Here's the drawing with two shaded views (mm, measured from the low corner). I have some questions. A direction names the side the tool comes from. Give positions to 0.01 mm unless a question says otherwise; leave off trailing zeros. Loops run counter-clockwise (first coordinate to the right, second up) from the corner with the lowest first, then second, coordinate; pieces in that order, holes last. Notation, with made-up numbers: M -21,-31.75 L 19,-31.75 A13 cw 19,-23.75 Z; hole C 28.25,21.5 d8. An arc over 180 degrees is marked long. Use a Markdown table: item, result. Add a question column.
1) Suppose I cut it at D-D on z = 2. List the corners of the cut face in (x, y) for me (3 decimals).
2) Suppose I cut it at C-C on z = 7. List the corners of the cut face in (x, y) for me, and give its area (3 significant figures).
3) If I drill on line 1 along X through (y, z) = (36, 10.25); line 2 along Z through (x, y) = (8, 28.5); line 3 along Y through (x, z) = (38.8, 6), over which ranges is the centre line in solid material (lowest first)? Write a range as [from, to].
4) Suppose I cut it at A-A on y = 30. List the corners of the cut face in (x, z) for me (3 decimals), and give its area (3 significant figures).
5) Which directions (+Z, -Z, +X, -X, +Y, -Y) give clear straight access to the entire face, cutting with the end or side of a thin tool? Please do the marked faces 1, 2 and 3.
6) We'd pull the mould along X, two halves only. Please class the marked faces 4, 5 and 6: +X half, -X half, draft (parallel to the pull), parting line (faces both ways), or undercut.
7) Suppose I cut it at B-B on x = 30. List the corners of the cut face in (y, z) for me.
8) Will these pins go through, and if not, where does the flat tip stop? pin 1 Ø13.5 at (x, y) = (38.8, 30) entering from +Z; pin 2 Ø1 at (x, z) = (42.5, 4.5) entering from -Y; pin 3 Ø1.5 at (x, y) = (8, 29.5) entering from -Z.
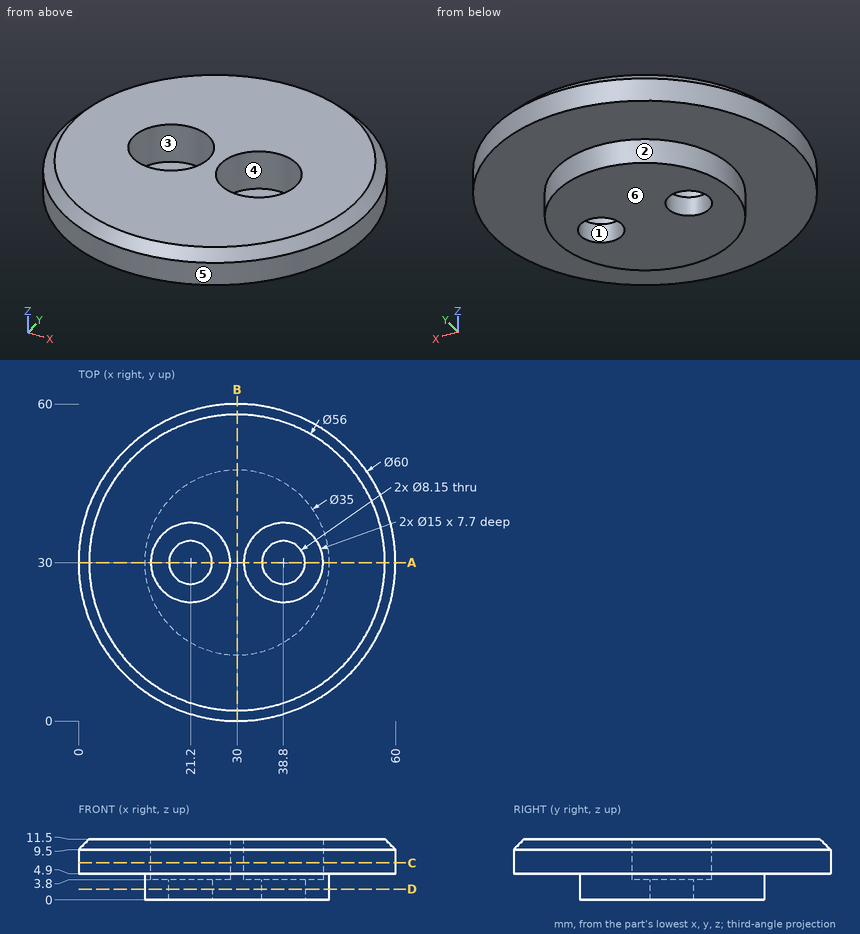
Answer block:
| question | item | result |
|---|---|---|
| 1 | outline | C 30,30 d35; hole C 21.2,30 d8.15; hole C 38.8,30 d8.15 |
| 2 | outline | C 30,30 d60; hole C 21.2,30 d15; hole C 38.8,30 d15 |
| 2 | area | 2,470 mm^2 |
| 3 | line 1 | x = [1.37, 16.7], [25.7, 34.3], [43.3, 58.63] |
| 3 | line 2 | z = [4.9, 11.5] |
| 3 | line 3 | y = [1.32, 22.5], [37.5, 58.68] |
| 4 | outline | M 0,4.9 L 12.5,4.9 L 12.5,0 L 17.125,0 L 17.125,3.8 L 13.7,3.8 L 13.7,11.5 L 2,11.5 L 0,9.5 Z; M 25.275,0 L 34.725,0 L 34.725,3.8 L 31.3,3.8 L 31.3,11.5 L 28.7,11.5 L 28.7,3.8 L 25.275,3.8 Z; M 42.875,0 L 47.5,0 L 47.5,4.9 L 60,4.9 L 60,9.5 L 58,11.5 L 46.3,11.5 L 46.3,3.8 L 42.875,3.8 Z |
| 4 | area | 271 mm^2 |
| 5 | face 1 | +Z, -Z |
| 5 | face 2 | -Z |
| 5 | face 3 | +Z |
| 6 | face 4 | undercut |
| 6 | face 5 | parting line |
| 6 | face 6 | draft |
| 7 | outline | M 0,4.9 L 12.5,4.9 L 12.5,0 L 47.5,0 L 47.5,4.9 L 60,4.9 L 60,9.5 L 58,11.5 L 2,11.5 L 0,9.5 Z |
| 8 | pin 1 | stops at z = 3.8 |
| 8 | pin 2 | stops at y = 2.59 |
| 8 | pin 3 | stops at z = 4.9 |
